Autodesk Inventor part; units mm, degrees
ref_plane "YZ Plane" through (0, 0, 0) normal (1, 0, 0) x (0, 1, 0)
ref_plane "XZ Plane" through (0, 0, 0) normal (0, 1, 0) x (-1, 0, 0)
ref_plane "XY Plane" through (0, 0, 0) normal (0, 0, 1) x (1, 0, 0)
sketch "スケッチ1" plane through (0, 0, 0) normal (0, 0, 1) x (1, 0, 0)
  circle A0 centre (0, 0) radius 3
  circle A1 centre (0, 0) radius 1.5
  dimension "d0" = 6
  dimension "d1" = 3
extrude "押し出し1" add sketch "スケッチ1" along normal blind 10
fillet "フィレット1" radius 0.3 1 edges at (-3, 0, 10)
fillet "フィレット2" radius 0.3 1 edges at (-3, 0, 0)
thread "ねじ1"
properties part number "スペーサーM3L10黄銅" material "アルミニウム 2014-T4"
For this review, take the finished solid that the model builds, in its own axes (mm). Round coordinates to 2 decimals unless told otherwise and drop trailing zeros. Write each loop counter-clockwise with the first axis right and the second up, starting at its lowest first coordinate (ties: lowest second). Pieces come first, ordered by that corner, then holes. Notation, with made-up numbers: (23, 57) - (57, 57) arc R27 cw to (57, 85) - close; hole circle Ø1 at (79.5, 43). An arc over 180 degrees is marked (long way). Put each result on its own line as item: value.
Q1. We need section A-A (x = 0). Give the boundary of the cut face in (y, z).
Solved:
outline: (-3, 0.3) arc R0.3 ccw to (-2.7, 0) - (-1.5, 0) - (-1.5, 10) - (-2.7, 10) arc R0.3 ccw to (-3, 9.7) - close; (1.5, 0) - (2.7, 0) arc R0.3 ccw to (3, 0.3) - (3, 9.7) arc R0.3 ccw to (2.7, 10) - (1.5, 10) - close
Q2. Wall thickness on probe 1 along Y at (x, z) = (0, 6.25); probe 2 along Y at (x, z) = (1.25, 7); probe 3 along X at (y, z) = (0.5, 6.5): over which ranges is each line inside the solid? List them lowest first.
Solved:
probe 1: y = -3 to -1.5, 1.5 to 3
probe 2: y = -2.73 to -0.83, 0.83 to 2.73
probe 3: x = -2.96 to -1.41, 1.41 to 2.96
Q3. Insertion check: pin 1 Ø2 at (x, y) = (1, -2) entering from -Z; pin 2 Ø2 at (y, z) = (-2, 9) entering from +X. Each pin has a flat end and moves straight along its axis. Give the tip position at first contact, or say it passes through.
Solved:
pin 1: stops at z = 0
pin 2: stops at x = 2.83
Q4. We need section C-C (z = 1.5). Give the boundary of the cut face in (x, y), and give its area (3 significant figures).
Solved:
outline: circle Ø6 at (0, 0); hole circle Ø3 at (0, 0)
area: 21.2 mm2
Q5. Mouldability with a two-part tool opening along X and no side actions: class faces 1 (the face through (-3, 0, 5)), 2 (the face through (1.2, -1.2, 10)), 3 (the face through (-1.5, -0.07, 4.93)) as released by +X, released by -X, zero draft, split by the parting line, or undercut.
Solved:
face 1: split by the parting line
face 2: zero draft
face 3: undercut
